```python
from build123d import *

# Parameters (mm, degrees)
SKETCH_1_W          = 23.5
SKETCH_1_H          = 41.5
EXTRUDE_1_DEPTH     = 15
SKETCH_2_W          = 5
SKETCH_2_H          = 18.5
CUT_EXTRUDE_1_DEPTH = 10
SKETCH_3_W          = 5
SKETCH_3_H          = 12.5
CUT_EXTRUDE_2_DEPTH = 6
SKETCH_4_R          = 1.5
CUT_EXTRUDE_3_DEPTH = 6


with BuildPart() as part:
    # 草图1 → 凸台-拉伸1 (new body)
    with BuildSketch(Plane.XY):
        Rectangle(SKETCH_1_W, SKETCH_1_H)
    extrude(amount=EXTRUDE_1_DEPTH)

    # 草图2 → 切除-拉伸1 (cut)
    with BuildSketch(Plane.XY.offset(15)):
        with Locations((-9.25, 11.5)):
            Rectangle(SKETCH_2_W, SKETCH_2_H)
        with Locations((9.25, 11.5)):
            Rectangle(SKETCH_2_W, SKETCH_2_H)
    extrude(amount=-CUT_EXTRUDE_1_DEPTH, mode=Mode.SUBTRACT)

    # 草图3 → 切除-拉伸2 (cut, through all)
    with BuildSketch(Plane.XY.offset(5)):
        with Locations((-9.25, 14.5)):
            Rectangle(SKETCH_3_W, SKETCH_3_H)
        with Locations((9.25, 14.5)):
            Rectangle(SKETCH_3_W, SKETCH_3_H)
    extrude(amount=-CUT_EXTRUDE_2_DEPTH, mode=Mode.SUBTRACT)

    # 草图4 → 切除-拉伸3 (cut, through all)
    with BuildSketch(Plane.XY.offset(5)):
        with Locations((-9.75, 5.25)):
            Circle(SKETCH_4_R)
        with Locations((9.75, 5.25)):
            Circle(SKETCH_4_R)
    extrude(amount=-CUT_EXTRUDE_3_DEPTH, mode=Mode.SUBTRACT)


solid = part.part
```
Here's how the part is built. I have some questions about the finished solid (model axes, mm). A direction names the side the tool comes from. Round coordinates to 2 decimals unless told otherwise and drop trailing zeros. Loops run counter-clockwise (first coordinate to the right, second up) from the corner with the lowest first, then second, coordinate; pieces in that order, holes last. Notation, with made-up numbers: (-39, -20) -> (13, -20) arc R8 ccw to (13, -7) -> close; hole circle Ø7 at (54.25, 46). An arc over 180 degrees is marked (long way). Answer as CSV lines item,"result".
1. For pin 1 (2 mm diameter, centred on x = -9.5, z = 12, fed in from +Y); pin 2 (8 mm diameter, centred on x = -9.5, y = 10, fed in from +Z); pin 3 (1.5 mm diameter, centred on x = 10.5, z = 2, fed in from +Y); pin 4 (2.5 mm diameter, centred on x = -9.5, y = 4.5, fed in from +Z), each with a flat end and sliding along its axis, tell me the tip position at first contact or that it passes through.
Final values:
pin 1,"stops at y = 2.25"
pin 2,"stops at z = 15"
pin 3,"stops at y = 8.25"
pin 4,"stops at z = 5"
2. If we section it at C-C on y = 5.25: Please give me the cut outline in (x, z).
Final values:
outline,"(-11.75, 0) -> (-11.25, 0) -> (-11.25, 5) -> (-11.75, 5) -> close; (-8.25, 0) -> (8.25, 0) -> (8.25, 5) -> (6.75, 5) -> (6.75, 15) -> (-6.75, 15) -> (-6.75, 5) -> (-8.25, 5) -> close; (11.25, 0) -> (11.75, 0) -> (11.75, 5) -> (11.25, 5) -> close"
3. Which directions (+Z, -Z, +X, -X, +Y, -Y) give clear straight access to the entire face, cutting with the end or side of a thin tool? Please do faces 1 (the face through (-9, 2.25, 10)), 2 (the face through (-9, 8.25, 3)), 3 (the face through (8, 5, 5)), 4 (the face through (0, -20.75, 7)), 5 (the face through (9, 8.25, 3)).
Final values:
face 1,"+Z, -X, +Y"
face 2,"+Z, -Z, -X, +Y"
face 3,"+Z, +X, +Y"
face 4,"+Z, -Z, +X, -X, -Y"
face 5,"+Z, -Z, +X, +Y"
4. If we section it at A-A on z = 2.75: Please give me the cut outline in (x, y), plus the area to 3 significant figures.
Final values:
outline,"(-11.75, -20.75) -> (11.75, -20.75) -> (11.75, 8.25) -> (6.75, 8.25) -> (6.75, 20.75) -> (-6.75, 20.75) -> (-6.75, 8.25) -> (-11.75, 8.25) -> close; hole circle Ø3 at (-9.75, 5.25); hole circle Ø3 at (9.75, 5.25)"
area,"836 mm^2"
5. If I drill on L1, parallel to Y at x = -9.75, z = 1.4; L2, parallel to Z at x = 8.25, y = 4; L3, parallel to X at y = 3.5, z = 13.5, over which ranges is the centre line in solid material (lowest first)?
Final values:
L1,"y = -20.75 to 3.75, 6.75 to 8.25"
L2,"z = 0 to 5"
L3,"x = -6.75 to 6.75"
6. If we section it at B-B on x = -9.75: Please give me the cut outline in (y, z).
Final values:
outline,"(-20.75, 0) -> (3.75, 0) -> (3.75, 5) -> (2.25, 5) -> (2.25, 15) -> (-20.75, 15) -> close; (6.75, 0) -> (8.25, 0) -> (8.25, 5) -> (6.75, 5) -> close"
7. If we section it at D-D on z = 5.75: Please give me the cut outline in (x, y), plus the area to 3 significant figures.
Final values:
outline,"(-11.75, -20.75) -> (11.75, -20.75) -> (11.75, 2.25) -> (6.75, 2.25) -> (6.75, 20.75) -> (-6.75, 20.75) -> (-6.75, 2.25) -> (-11.75, 2.25) -> close"
area,"790 mm^2"
8. Thinking about a two-plate mould opening in X: for faces 6 (the face through (0, -4, 15)), 7 (the face through (8.25, 5.32, 2.54)), 8 (the face through (11.75, -10, 7)), 9 (the face through (-11.75, -10, 7)), which applies, released by +X, released by -X, zero draft, split by the parting line, or undercut?
Final values:
face 6,"zero draft"
face 7,"undercut"
face 8,"released by +X"
face 9,"released by -X"
